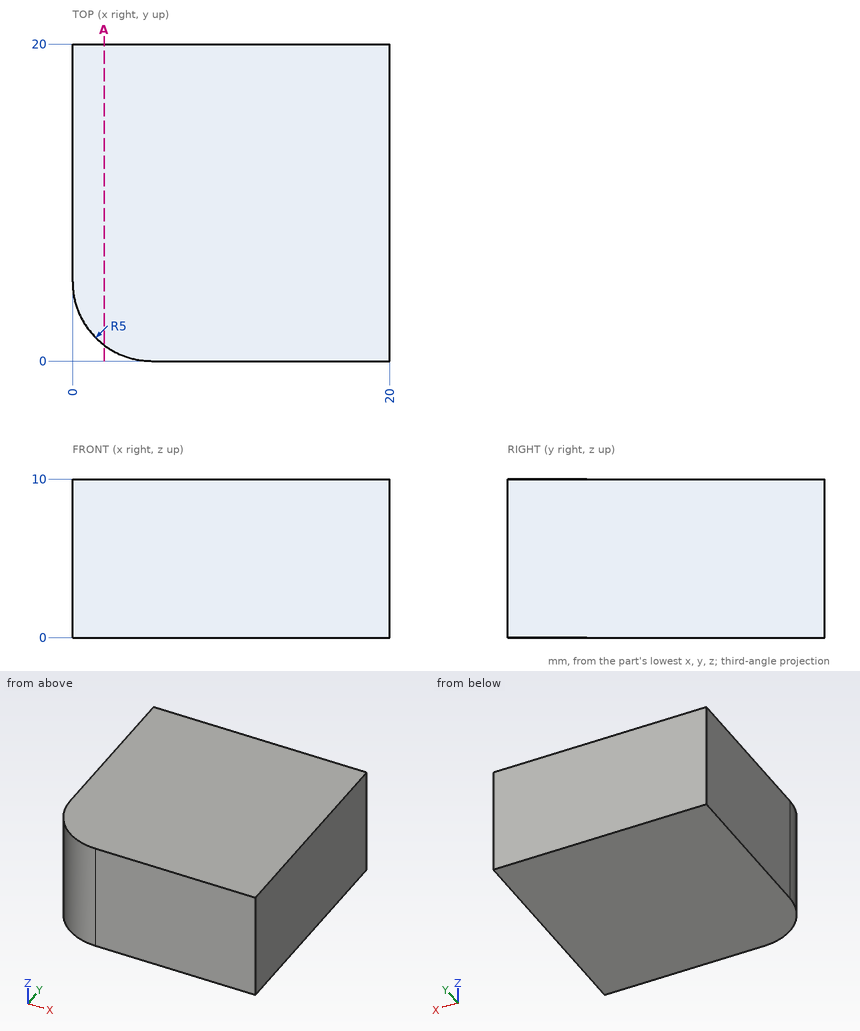
The drawing under review shows one solid part. Ordinate dimensions are in mm from its lowest x, y, z. Round coordinates to 2 decimals unless told otherwise and drop trailing zeros. Write each loop counter-clockwise with the first axis right and the second up, starting at its lowest first coordinate (ties: lowest second). Pieces come first, ordered by that corner, then holes. Notation, with made-up numbers: (1, -38.75) - (55, -38.75) arc R29 ccw to (55, 0.25) - close; hole circle Ø9 at (-27.75, 42.5). An arc over 180 degrees is marked (long way). One line per question, with ' | ' between items.
Item 1: For P1, Ø1, axis at y = 4, z = 5, coming from the -X side; P2, Ø6, axis at x = 9.5, y = 17.5, coming from the -Z side, all flat-tipped, find the tip position at first contact; note any pin that passes through.
Resolved:
P1: stops at x = 0.03 | P2: stops at z = 0
Item 2: Add section A-A, the plane x = 2. Give the boundary of the cut face in (y, z).
Resolved:
outline: (1, 0) - (20, 0) - (20, 10) - (1, 10) - close
Item 3: To check wall thickness, follow probe 1 along Y at (x, z) = (4.75, 2.25); probe 2 along X at (y, z) = (1.25, 4.25). State the ranges of each line that lie inside material, in increasing order.
Resolved:
probe 1: y = 0.01 to 20 | probe 2: x = 1.69 to 20
